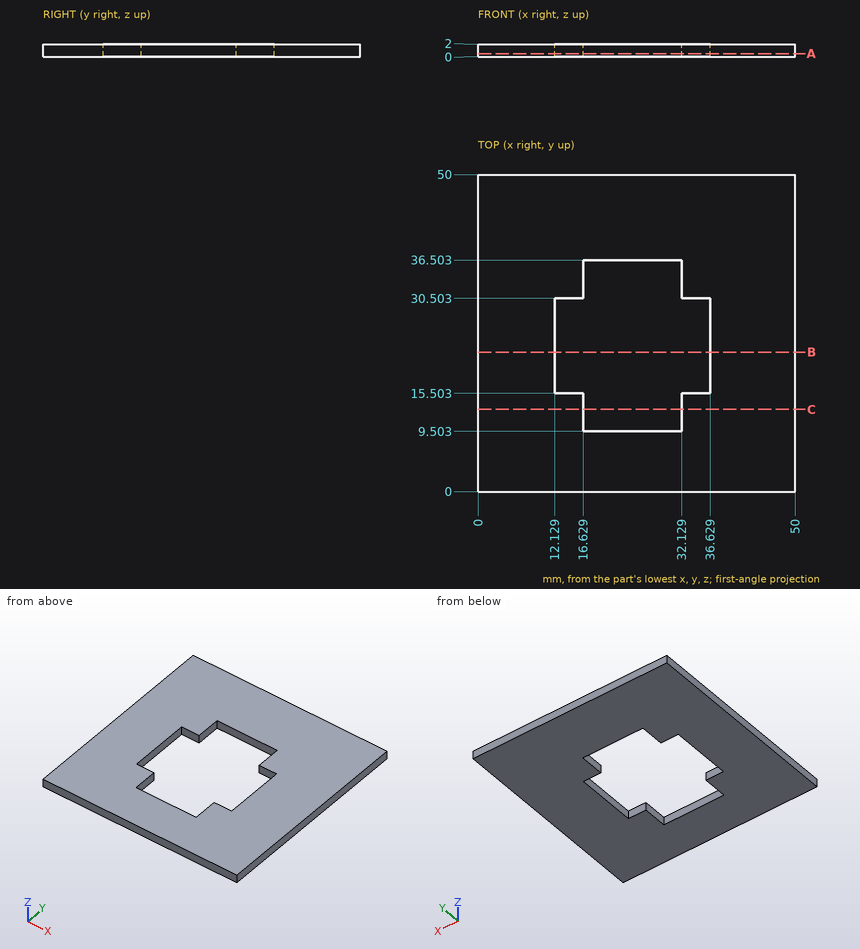
Answer from the drawing. Dimensions are ordinates in mm from the lowest x, y and z of the part. Give positions to 0.01 mm unless a question says otherwise; leave off trailing zeros. Loops run counter-clockwise (first coordinate to the right, second up) from the corner with the lowest first, then second, coordinate; pieces in that order, holes last. Notation, with made-up numbers: (34.5, 17.25) -> (91.5, 17.25) arc R24 ccw to (91.5, 54.25) -> close; hole circle Ø11 at (-19, 86). An arc over 180 degrees is marked (long way). Use a Markdown table: item, result.
Q1. Find the intervals of material crossed by line 1 along Y through (x, z) = (13, 0.35); line 2 along Y through (x, z) = (22.5, 1.55); line 3 along X through (y, z) = (35, 1.4), in increasing order.
Solved:
| item | result |
|---|---|
| line 1 | y = 0 to 15.5, 30.5 to 50 |
| line 2 | y = 0 to 9.5, 36.5 to 50 |
| line 3 | x = 0 to 16.63, 32.13 to 50 |
Q2. Section B-B, the plane y = 22 is taken. Determine the outline of the cut face in (x, z).
Solved:
| item | result |
|---|---|
| outline | (0, 0) -> (12.13, 0) -> (12.13, 2) -> (0, 2) -> close; (36.63, 0) -> (50, 0) -> (50, 2) -> (36.63, 2) -> close |
Q3. Section C-C, the plane y = 13 is taken. Determine the outline of the cut face in (x, z).
Solved:
| item | result |
|---|---|
| outline | (0, 0) -> (16.63, 0) -> (16.63, 2) -> (0, 2) -> close; (32.13, 0) -> (50, 0) -> (50, 2) -> (32.13, 2) -> close |
Q4. Section A-A, the plane z = 0.5 is taken. Determine the outline of the cut face in (x, y).
Solved:
| item | result |
|---|---|
| outline | (0, 0) -> (50, 0) -> (50, 50) -> (0, 50) -> close; hole (12.13, 15.5) -> (16.63, 15.5) -> (16.63, 9.5) -> (32.13, 9.5) -> (32.13, 15.5) -> (36.63, 15.5) -> (36.63, 30.5) -> (32.13, 30.5) -> (32.13, 36.5) -> (16.63, 36.5) -> (16.63, 30.5) -> (12.13, 30.5) -> close |
